from build123d import *

# Parameters (mm, degrees)
EXTRUDE_1_DEPTH      = 3.5
EXTRUDE_1_DEPTH_BACK = 11.7
SKETCH_1_W           = 53
SKETCH_1_H           = 48
CUT_EXTRUDE_START    = -1.6
CUT_EXTRUDE_1_DEPTH  = 1.6
CUT_EXTRUDE_2_DEPTH  = 2
SKETCH_5_R           = 2
CUT_EXTRUDE_3_DEPTH  = 0.8
FILLET_2_R           = 1.5
FILLET_1_R           = 3
CUT_EXTRUDE_4_DEPTH  = 38.15185056
CUT_EXTRUDE_6_REACH  = 58.064
CUT_EXTRUDE_8_REACH  = 56.752
SKETCH_8_W           = 2.9
SKETCH_8_H           = 1.5
CUT_EXTRUDE_7_DEPTH  = 2.5
EXTRUDE_2_DEPTH      = 1.5


# Read off the part's stored shape, not the designer's step: 切除-旋转2
with BuildPart() as part:
    # 草图1 → 凸台-拉伸1 (new, two sides: drawn at the far end of the back side and taken through both)
    with BuildSketch(Plane.XY.offset(-EXTRUDE_1_DEPTH_BACK)):
        Rectangle(SKETCH_1_W, SKETCH_1_H)
    extrude(amount=EXTRUDE_1_DEPTH + EXTRUDE_1_DEPTH_BACK)

    # 草图2 → 切除-拉伸1 (cut)
    with BuildSketch(Plane.XY.offset(CUT_EXTRUDE_START)):
        Polygon((-25.04302926, 22.538726334), (-25.04302926, -22.461273666), (24.95697074, -22.461273666), (24.95697074, 19.538726334), (21.95697074, 22.538726334), align=None)
    extrude(amount=CUT_EXTRUDE_1_DEPTH, mode=Mode.SUBTRACT)

    # 草图3 → 切除-拉伸2 (cut)
    with BuildSketch(Plane.XY):
        Polygon((-23.04302926, 20.538726334), (-23.04302926, -20.461273666), (22.95697074, -20.461273666), (22.95697074, 18.710299209), (21.128543615, 20.538726334), align=None)
    extrude(amount=CUT_EXTRUDE_2_DEPTH, mode=Mode.SUBTRACT)

    # 草图5 → 切除-拉伸3 (cut)
    with BuildSketch(Plane(origin=(0, 0, 2), x_dir=(-1, 0, 0), z_dir=(0, 0, -1))):
        with Locations((0, 10.596648324)):
            Circle(SKETCH_5_R)
        with Locations((-4.257893586, 14.765199175)):
            Circle(SKETCH_5_R)
        with Locations((-9.74067964, 16.855011719)):
            Circle(SKETCH_5_R)
        with Locations((-15.42583133, 15.403354164)):
            Circle(SKETCH_5_R)
        with Locations((-19.235519258, 10.94078346)):
            Circle(SKETCH_5_R)
        with Locations((-19.777365172, 5.098295771)):
            Circle(SKETCH_5_R)
        with Locations((-16.859691363, 0.004679646)):
            Circle(SKETCH_5_R)
        with Locations((-12.644768522, -4.210243195)):
            Circle(SKETCH_5_R)
        with Locations((-8.429845681, -8.425166036)):
            Circle(SKETCH_5_R)
        with Locations((-4.21492284, -12.640088876)):
            Circle(SKETCH_5_R)
        with Locations((0, -16.855011717)):
            Circle(SKETCH_5_R)
        with Locations((4.21492284, -12.640088877)):
            Circle(SKETCH_5_R)
        with Locations((8.429845681, -8.425166037)):
            Circle(SKETCH_5_R)
        with Locations((12.644768522, -4.210243196)):
            Circle(SKETCH_5_R)
        with Locations((16.859691363, 0.004679645)):
            Circle(SKETCH_5_R)
        with Locations((19.777365172, 5.09829577)):
            Circle(SKETCH_5_R)
        with Locations((19.235519258, 10.940783459)):
            Circle(SKETCH_5_R)
        with Locations((15.425831331, 15.403354163)):
            Circle(SKETCH_5_R)
        with Locations((9.740679641, 16.855011718)):
            Circle(SKETCH_5_R)
        with Locations((4.257893587, 14.765199175)):
            Circle(SKETCH_5_R)
    extrude(amount=-CUT_EXTRUDE_3_DEPTH, mode=Mode.SUBTRACT)

    # 圆角2
    fillet_2_edges = [part.edges().sort_by_distance(p)[0] for p in [
        (24.95697074, -22.461273666, -0.8),
        (-25.04302926, -22.461273666, -0.8),
        (-25.04302926, 22.538726334, -0.8),
        (-23.04302926, 20.538726334, 1),
        (-23.04302926, -20.461273666, 1),
        (22.95697074, -20.461273666, 1),
    ]]
    fillet(fillet_2_edges, radius=FILLET_2_R)

    # 圆角1
    fillet_1_edges = [part.edges().sort_by_distance(p)[0] for p in [
        (26.5, 24, -4.1),
        (-26.5, 24, -4.1),
        (-26.5, -24, -4.1),
        (26.5, -24, -4.1),
    ]]
    fillet(fillet_1_edges, radius=FILLET_1_R)

    # 草图6 → 切除-拉伸4 (cut, through all)
    with BuildSketch(Plane.XY.offset(-1.6)):
        with BuildLine():
            Line((-23.54302926, -22.461273666), (23.45697074, -22.461273666))
            ThreePointArc((23.45697074, -22.461273666), (24.517630912, -22.021933838), (24.95697074, -20.961273666))
            Line((24.95697074, -20.961273666), (24.95697074, 21.038726334))
            ThreePointArc((24.95697074, 21.038726334), (24.517630912, 22.099386506), (23.45697074, 22.538726334))
            Line((23.45697074, 22.538726334), (-23.54302926, 22.538726334))
            ThreePointArc((-23.54302926, 22.538726334), (-24.603689432, 22.099386506), (-25.04302926, 21.038726334))
            Line((-25.04302926, 21.038726334), (-25.04302926, -20.961273666))
            ThreePointArc((-25.04302926, -20.961273666), (-24.603689432, -22.021933838), (-23.54302926, -22.461273666))
        make_face()
    extrude(amount=-CUT_EXTRUDE_4_DEPTH, mode=Mode.SUBTRACT)

    # 草图7 → 切除-拉伸6 (cut, up to next)
    with BuildSketch(Plane.XZ.offset(24), mode=Mode.PRIVATE) as cut_extrude_6_sk1:
        with BuildLine():
            Line((2.9, -2.8), (-2.9, -2.8))
            ThreePointArc((-2.9, -2.8), (-5, -4.9), (-2.9, -7))
            Line((-2.9, -7), (2.9, -7))
            ThreePointArc((2.9, -7), (5, -4.9), (2.9, -2.8))
        make_face()
    cut_extrude_6_tool1 = extrude(cut_extrude_6_sk1.sketch, amount=-CUT_EXTRUDE_6_REACH, mode=Mode.PRIVATE) & part.part
    add(cut_extrude_6_tool1.solids().sort_by_distance((0, -24, -4.9))[0], mode=Mode.SUBTRACT)

    # 草图8 → 切除-拉伸8 (cut, up to next)
    with BuildSketch(Plane.XZ.offset(22.461273666), mode=Mode.PRIVATE) as cut_extrude_8_sk1:
        with Locations((-16.99302926, -2.35)):
            Rectangle(SKETCH_8_W, SKETCH_8_H)
    cut_extrude_8_tool1 = extrude(cut_extrude_8_sk1.sketch, amount=CUT_EXTRUDE_8_REACH, mode=Mode.PRIVATE) & part.part
    add(cut_extrude_8_tool1.solids().sort_by_distance((-16.993029, -22.461274, -2.35))[0], mode=Mode.SUBTRACT)

    # 草图11 → 切除-拉伸7 (cut, symmetric)
    with BuildSketch(Plane.ZY.offset(16.99302926)):
        with BuildLine():
            Line((-1.6, -22.961273666), (-3.1, -22.961273666))
            ThreePointArc((-3.1, -22.961273666), (-4.339097696, -23.233488179), (-5.35, -24))
            Line((-5.35, -24), (0.65, -24))
            ThreePointArc((0.65, -24), (-0.360902304, -23.233488179), (-1.6, -22.961273666))
        make_face()
    extrude(amount=CUT_EXTRUDE_7_DEPTH, both=True, mode=Mode.SUBTRACT)

    # 草图12 → 切除-旋转1 (revolve, cut)
    with BuildSketch(Plane(origin=(-19.49302926, 0, 0), x_dir=(0, 0, -1), z_dir=(1, 0, 0))):
        with BuildLine():
            Line((-0.65, -24), (5.35, -24))
            ThreePointArc((5.35, -24), (4.339097696, -23.233488179), (3.1, -22.961273666))
            Line((3.1, -22.961273666), (1.6, -22.961273666))
            ThreePointArc((1.6, -22.961273666), (0.360902304, -23.233488179), (-0.65, -24))
        make_face()
    revolve(axis=Axis((-19.49302926, -24, 0.65), (0, 0, -1)), mode=Mode.SUBTRACT)

    # 切除-旋转2 outline → 切除-旋转2 (revolve, cut)
    with BuildSketch(Plane(origin=(-14.49302926, -24, 0), x_dir=(1, 0, 0), z_dir=(0, -1, 0))):
        with BuildLine():
            add(Edge.make_bspline(
                [(1.038726334, -3.1), (1.038726334, -4.464767199), (0, -5.35)],
                knots=[0, 0, 0, 0.865009582, 0.865009582, 0.865009582], degree=2, weights=[1, 0.907918725, 1]))
            Line((1.038726334, -3.1), (1.038726334, -1.6))
            add(Edge.make_bspline(
                [(0, 0.65), (1.038726334, -0.235232801), (1.038726334, -1.6)],
                knots=[5.418175725, 5.418175725, 5.418175725, 6.283185307, 6.283185307, 6.283185307], degree=2, weights=[1, 0.907918725, 1]))
            Line((0, 0.65), (0, -5.35))
        make_face()
    revolve(axis=Axis((-14.49302926, -24, 0), (0, 0, 1)), mode=Mode.SUBTRACT)

    # 草图14 → 凸台-拉伸2 (add)
    with BuildSketch(Plane(origin=(0, 0, -11.7), x_dir=(-1, 0, 0), z_dir=(0, 0, -1))):
        with BuildLine():
            Line((-26.5, 21), (-26.5, -21))
            ThreePointArc((-26.5, -21), (-25.621320344, -23.121320344), (-23.5, -24))
            Line((-23.5, -24), (23.5, -24))
            ThreePointArc((23.5, -24), (25.621320344, -23.121320344), (26.5, -21))
            Line((26.5, -21), (26.5, 21))
            ThreePointArc((26.5, 21), (25.621320344, 23.121320344), (23.5, 24))
            Line((23.5, 24), (-23.5, 24))
            ThreePointArc((-23.5, 24), (-25.621320344, 23.121320344), (-26.5, 21))
        make_face()
    extrude(amount=-EXTRUDE_2_DEPTH)


solid = part.part
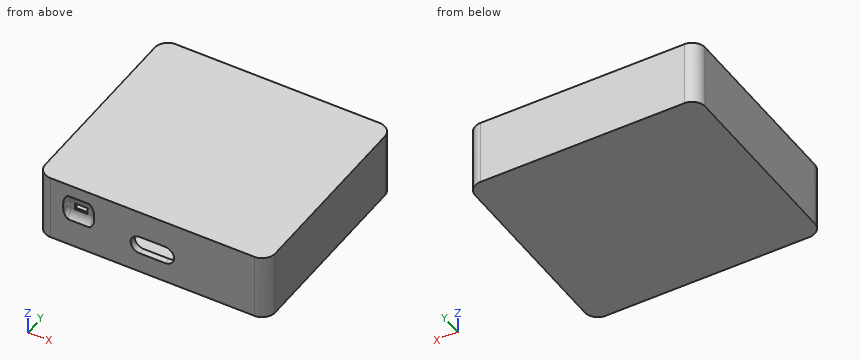
Could you check a few things on this model? Use its own coordinates, in mm. Give positions to 0.01 mm unless a question says otherwise; leave off trailing zeros. Loops run counter-clockwise (first coordinate to the right, second up) from the corner with the lowest first, then second, coordinate; pieces in that order, holes last. Notation, with made-up numbers: (63, 18) -> (102, 18) arc R21 ccw to (102, 32) -> close; hole circle Ø6 at (48.5, 56.5). An arc over 180 degrees is marked (long way). Answer as CSV lines item,"result". Start each with the question number.
(1) If we section it at D-D on y = 14: Write out the boundary of the cut face in (x, z).
(2) If we section it at A-A on y = -12: Write out the boundary of the cut face in (x, z).
(3) I need wall thicknesses on probe 1 along X at (y, z) = (1.5, -8.25); probe 2 along Z at (x, y) = (-5, 11); probe 3 along Y at (x, z) = (0.5, 1). Which ranges of each line are inside material? Lowest first, please.
(4) If we section it at B-B on x = 8.5: Write out the boundary of the cut face in (y, z), then the cut area to 3 significant figures.
(5) If we section it at C-C on x = 0: Write out the boundary of the cut face in (y, z), then the cut area to 3 significant figures.
Computed:
1,outline,"(-26.5, -11.7) -> (26.5, -11.7) -> (26.5, 3.5) -> (-26.5, 3.5) -> close; hole (-25.04, -10.2) -> (24.96, -10.2) -> (24.96, 0) -> (22.96, 0) -> (22.96, 2) -> (16.85, 2) -> (16.85, 2.8) -> (14, 2.8) -> (14, 2) -> (6.11, 2) -> (6.11, 2.8) -> (2.41, 2.8) -> (2.41, 2) -> (-2.41, 2) -> (-2.41, 2.8) -> (-6.11, 2.8) -> (-6.11, 2) -> (-14, 2) -> (-14, 2.8) -> (-16.85, 2.8) -> (-16.85, 2) -> (-23.04, 2) -> (-23.04, 0) -> (-25.04, 0) -> close"
2,outline,"(-26.5, -11.7) -> (26.5, -11.7) -> (26.5, 3.5) -> (-26.5, 3.5) -> close; hole (-25.04, -10.2) -> (24.96, -10.2) -> (24.96, 0) -> (22.96, 0) -> (22.96, 2) -> (6.11, 2) -> (6.11, 2.8) -> (2.32, 2.8) -> (2.32, 2) -> (-2.32, 2) -> (-2.32, 2.8) -> (-6.11, 2.8) -> (-6.11, 2) -> (-23.04, 2) -> (-23.04, 0) -> (-25.04, 0) -> close"
3,probe 1,"x = -26.5 to -25.04, 24.96 to 26.5"
3,probe 2,"z = -11.7 to -10.2, 2 to 3.5"
3,probe 3,"y = -24 to -20.46, 20.54 to 24"
4,outline,"(-24, -11.7) -> (24, -11.7) -> (24, 3.5) -> (-24, 3.5) -> close; hole (-22.46, -10.2) -> (22.54, -10.2) -> (22.54, 0) -> (20.54, 0) -> (20.54, 2) -> (18.42, 2) -> (18.42, 2.8) -> (15.29, 2.8) -> (15.29, 2) -> (-6.43, 2) -> (-6.43, 2.8) -> (-10.42, 2.8) -> (-10.42, 2) -> (-20.46, 2) -> (-20.46, 0) -> (-22.46, 0) -> close"
4,area,"183 mm2"
5,outline,"(-24, -11.7) -> (24, -11.7) -> (24, 3.5) -> (-24, 3.5) -> (-24, -2.8) -> (-22.46, -2.8) -> (-22.46, 0) -> (-20.46, 0) -> (-20.46, 2) -> (-18.86, 2) -> (-18.86, 2.8) -> (-14.86, 2.8) -> (-14.86, 2) -> (8.6, 2) -> (8.6, 2.8) -> (12.6, 2.8) -> (12.6, 2) -> (20.54, 2) -> (20.54, 0) -> (22.54, 0) -> (22.54, -10.2) -> (-22.46, -10.2) -> (-22.46, -7) -> (-24, -7) -> close"
5,area,"176 mm2"
